The drawing under review shows one solid part. Ordinate dimensions are in mm from its lowest x, y, z. A direction names the side the tool comes from. Coordinates: 2 decimals unless noted, no trailing zeros. Loops run counter-clockwise (first coordinate to the right, second up) from the corner with the lowest first, then second, coordinate; pieces in that order, holes last. Notation, with made-up numbers: M -20.75,-3 L 28.25,-3 A18 ccw 28.25,10 Z; hole C -14,31.5 d9. An arc over 180 degrees is marked long. Answer as CSV lines item,"result". Start each with the question number.
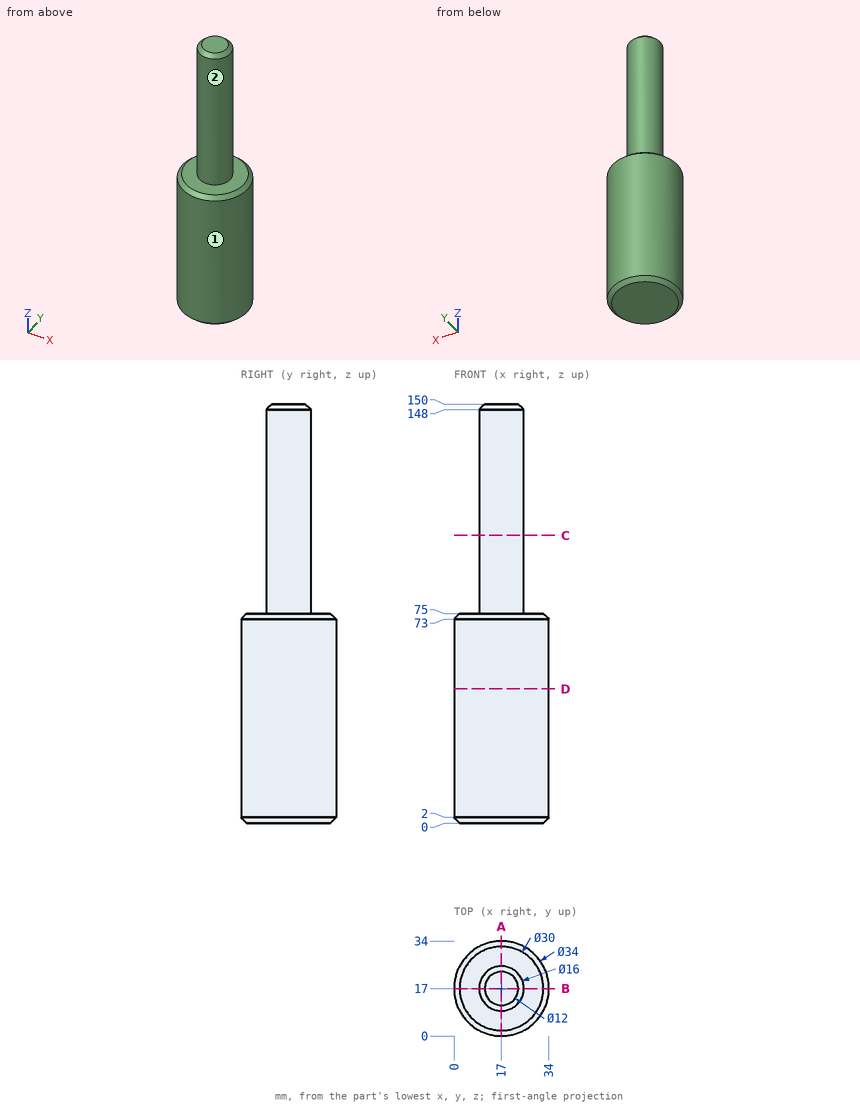
Item 1: For the marked faces 1 and 2, list the 3-axis set-ups (+Z, -Z, +X, -X, +Y, -Y) from which the entire face can be reached by the end or side of a thin tool; tool diameter is ignored.
Item 2: Add section C-C (z = 103). Give the boundary of the cut face in (x, y), plus the area to 3 significant figures.
Item 3: Add section A-A (x = 17). Give the boundary of the cut face in (y, z), plus the area to 3 significant figures.
Item 4: For line 1 along Z through (x, y) = (12, 24); line 2 along X through (y, z) = (16.5, 119); line 3 along Y through (x, z) = (16, 38.5), list the stretches that pass through material, from the lowest coordinate up. Write a range as from..to.
Item 5: For pin 1 (8 mm diameter, centred on x = 11, z = 63, fed in from -Y); pin 2 (1 mm diameter, centred on x = 12.5, z = 47.5, fed in from -Y); pin 3 (4 mm diameter, centred on y = 10.5, z = 88.5, fed in from +X); pin 4 (1.5 mm diameter, centred on x = 30.5, y = 4, fed in from -Z), all flat-tipped, find the tip position at first contact; note any pin that passes through.
Item 6: Add section D-D (z = 48). Give the boundary of the cut face in (x, y), plus the area to 3 significant figures.
Response:
1,face 1,"+Z, -Z"
1,face 2,"+Z"
2,outline,"C 17,17 d16"
2,area,"201 mm²"
3,outline,"M 0,2 L 2,0 L 32,0 L 34,2 L 34,73 L 32,75 L 25,75 L 25,148 L 23,150 L 11,150 L 9,148 L 9,75 L 2,75 L 0,73 Z"
3,area,"3,740 mm²"
4,line 1,"0..75"
4,line 2,"9.02..24.98"
4,line 3,"0.03..33.97"
5,pin 1,"y = 0.12"
5,pin 2,"y = 0.48"
5,pin 3,"x = 23.61"
5,pin 4,"through"
6,outline,"C 17,17 d34"
6,area,"908 mm²"
